from build123d import *

# Parameters (mm, degrees)
BOSS_EXTRUDE1_DEPTH = 100
FILLET1_R           = 50
CUT_EXTRUDE1_DEPTH  = 300


with BuildPart() as part:
    # Sketch1 → Boss-Extrude1 (new, symmetric)
    with BuildSketch(Plane(origin=(0, 0, 0), x_dir=(0, 0, -1), z_dir=(1, 0, 0))):
        with BuildLine():
            Line((-537.016574586, 60.497237569), (11.602209945, -135.082872928))
            Line((11.602209945, -135.082872928), (962.983425414, -135.082872928))
            ThreePointArc((962.983425414, -135.082872928), (1060.773480663, -37.29281768), (962.983425414, 60.497237569))
            Line((962.983425414, 60.497237569), (-537.016574586, 60.497237569))
        make_face()
    extrude(amount=BOSS_EXTRUDE1_DEPTH, both=True)

    # Fillet1
    fillet1_edges = [part.edges().sort_by_distance(p)[0] for p in [
        (-100, -135.082872928, -487.29281768),
        (-100, -37.29281768, 262.70718232),
        (-100, 60.497237569, -212.983425414),
        (100, -37.29281768, 262.70718232),
        (100, -135.082872928, -487.29281768),
        (100, -37.29281768, -1060.773480663),
        (100, 60.497237569, -212.983425414),
        (-100, -37.29281768, -1060.773480663),
    ]]
    fillet(fillet1_edges, radius=FILLET1_R)

    # Sketch2 → Cut-Extrude1 (cut)
    with BuildSketch(Plane.ZY.offset(100)):
        with BuildLine():
            Line((-240.278412459, 23.075070398), (-475.216763111, 23.075070398))
            ThreePointArc((-475.216763111, 23.075070398), (-490.247556178, 39.100328004), (-473.293494818, 53.075070398))
            Line((-473.293494818, 53.075070398), (-240.278412459, 23.075070398))
        make_face()
    extrude(amount=-CUT_EXTRUDE1_DEPTH, mode=Mode.SUBTRACT)


solid = part.part
Verification items for the finished model (mm, model axes). Coordinates: 2 decimals unless noted, no trailing zeros. Write each loop counter-clockwise with the first axis right and the second up, starting at its lowest first coordinate (ties: lowest second). Pieces come first, ordered by that corner, then holes. Notation, with made-up numbers: (-34.5, 87) -> (-16.5, 87) arc R30 cw to (-16.5, 123) -> close; hole circle Ø2 at (-1.75, 38.5). An arc over 180 degrees is marked (long way). One line per item, written item: value. Start each with the question number.
Q1. Thickness scan on L1, parallel to Y at x = -12.5, z = -447.5; L2, parallel to X at y = -80.5, z = 7; L3, parallel to Y at x = -51.5, z = -549. Record the ranges inside material, lowest first. Write a range as from..to.
Q2. Cross-section at C-C on z = -408. Enter the section's corners in (x, y).
Q3. Cross-section at A-A on z = -850.5. Enter the section's corners in (x, y).
Q4. Cross-section at B-B on x = -1. Enter the section's corners in (y, z), and give its area (3 significant figures).
Q5. Mould release check, pull along Z, two halves, no side actions. Record for faces 1 (the cylindrical face through (-1.377, 38.756, -490.266)), 2 (the flat face through (1, -135.083, -481)), 3 (the cylindrical face through (-84.964, -46.963, 193.121)): pulls with the +Z half, pulls with the -Z half, needs draft (parallel to the pull), parting line crosses it, or undercut.
Q6. Go/stop test with flat-tipped pins: P1, Ø6, axis at x = 29.5, y = -86, coming from the -Z side; P2, Ø5, axis at x = 70, z = -766.5, coming from the -Y side; P3, Ø1, axis at y = -114, z = -26, coming from the +X side. Record where each tip stops, or that it passes through.
Checked values:
1. L1: y = -135.08..23.08, 49.75..60.5
1. L2: x = -99.77..99.77
1. L3: y = -135.06..60.47
2. outline: (-100, -85.08) arc R50 ccw to (-50, -135.08) -> (50, -135.08) arc R50 ccw to (100, -85.08) -> (100, 10.5) arc R50 ccw to (98.39, 23.08) -> (-98.39, 23.08) arc R50 ccw to (-100, 10.5) -> close; (-86.5, 44.67) -> (86.5, 44.67) arc R50 ccw to (50, 60.5) -> (-50, 60.5) arc R50 ccw to start
3. outline: (-100, -85.08) arc R50 ccw to (-50, -135.08) -> (50, -135.08) arc R50 ccw to (100, -85.08) -> (100, 10.5) arc R50 ccw to (50, 60.5) -> (-50, 60.5) arc R50 ccw to (-100, 10.5) -> close
4. outline: (-135.08, -962.98) arc R97.79 ccw to (60.5, -962.98) -> (60.5, 537.02) -> (-135.08, -11.6) -> close; hole (23.08, -475.22) arc R15.06 ccw (long way) to (53.08, -473.29) -> (23.08, -240.28) -> close
4. area: 251,000 mm²
5. face 1: undercut
5. face 2: needs draft
5. face 3: pulls with the +Z half
6. P1: stops at z = -1049.43
6. P2: stops at y = -131.92
6. P3: stops at x = 91.14
